```python
from build123d import *

# Parameters (mm, degrees)
SKETCH1_W           = 20
SKETCH1_H           = 3
BOSS_EXTRUDE1_DEPTH = 3


with BuildPart() as part:
    # Sketch1 → Boss-Extrude1 (new body)
    # profile 1 of 3: a face of its own
    with BuildSketch(Plane.XY):
        Polygon((35, 40), (-35, 25), (-38, 25), (-38, 12.5), (-35, 12.5), (-35, -2.5), (-38, -2.5), (-38, -17.5), (-35, -17.5), (-35, -32.5), (-38, -32.5), (-38, -40), (-27.5, -40), (-7.5, -40), (7.5, -40), (27.5, -40), (38, -40), (38, -37.5), (35, -37.5), (35, -22.5), (38, -22.5), (38, -7.5), (35, -7.5), (35, 7.5), (38, 7.5), (38, 22.5), (35, 22.5), (35, 37.5), (38, 37.5), (38, 40), align=None)
        with BuildLine():
            ThreePointArc((-12.5, -28), (-17.5, -33), (-22.5, -28))
            Line((-22.5, -28), (-22.5, 12))
            ThreePointArc((-22.5, 12), (-17.5, 17), (-12.5, 12))
            Line((-12.5, 12), (-12.5, -28))
        make_face(mode=Mode.SUBTRACT)
        with BuildLine():
            ThreePointArc((-5, 17), (0, 22), (5, 17))
            Line((5, 17), (5, -28))
            ThreePointArc((5, -28), (0, -33), (-5, -28))
            Line((-5, -28), (-5, 17))
        make_face(mode=Mode.SUBTRACT)
        with BuildLine():
            ThreePointArc((22.5, -28), (17.5, -33), (12.5, -28))
            Line((12.5, -28), (12.5, 22))
            ThreePointArc((12.5, 22), (17.5, 27), (22.5, 22))
            Line((22.5, 22), (22.5, -28))
        make_face(mode=Mode.SUBTRACT)
    # profile 2 of 3: a face of its own
    with BuildSketch(Plane.XY):
        with Locations((17.5, -41.5)):
            Rectangle(SKETCH1_W, SKETCH1_H)
    # profile 3 of 3: a face of its own
    with BuildSketch(Plane.XY):
        with Locations((-17.5, -41.5)):
            Rectangle(SKETCH1_W, SKETCH1_H)
    extrude(amount=BOSS_EXTRUDE1_DEPTH)


solid = part.part
```
Geometry check sheet. Reference: the model listing, model coordinates, mm. A direction names the side the tool comes from. Give positions to 0.01 mm unless a question says otherwise; leave off trailing zeros. Order: outer loops, then holes, each group sorted by start corner. A loop starts at its lowest first (then second) coordinate and runs counter-clockwise, first axis right, second up.
1. Gauge pin test, flat ends, axial feed: pin 1 Ø1.5 at (y, z) = (5, 2) entering from +X; pin 2 Ø1.5 at (y, z) = (-24, 2) entering from -X; pin 3 Ø0.9 at (x, z) = (34, 1.5) entering from -Y. Record the tip position at first contact, or that the pin passes through.
2. Thickness scan on L1, parallel to X at y = -1, z = 1.45; L2, parallel to X at y = -21, z = 1.05; L3, parallel to X at y = 19.5, z = 1.2. Record the ranges inside material, lowest first.
3. Release check for a two-part mould opening along X. For faces 1 (the face through (-17.6, 17, 1.5)), 2 (the face through (36, -22.5, 1)), 3 (the face through (38, 39, 1)) record: pulls with the +X half, pulls with the -X half, needs draft (parallel to the pull), parting line crosses it, or undercut.
4. Access from +Z, -Z, +X, -X, +Y, -Y to the whole of each face (thin tool, end or side, straight path). Record for faces 4 (the face through (37, 22.5, 1)), 5 (the face through (33, -40, 1)), 6 (the face through (-22.5, -8, 1)).
5. Section check D-D, the plane x = 0. Enter the section's corners in (y, z).
6. Section check C-C, the plane z = 0.7. Give the number of separate pieces and of enclosed holes in the cut face, and give its area (3 significant figures).
7. Section check B-B, the plane x = 17.5. Enter the section's corners in (y, z), and give its area (4 significant figures).
8. Section check A-A, the plane y = -1.5. Enter the section's corners in (x, z).
Values follow:
1. pin 1: stops at x = 35
1. pin 2: stops at x = -35
1. pin 3: stops at y = -40
2. L1: x = -35 to -22.5, -12.5 to -5, 5 to 12.5, 22.5 to 35
2. L2: x = -35 to -22.5, -12.5 to -5, 5 to 12.5, 22.5 to 38
2. L3: x = -38 to -4.33, 4.33 to 12.5, 22.5 to 38
3. face 1: undercut
3. face 2: needs draft
3. face 3: pulls with the +X half
4. face 4: +Z, -Z, +X
4. face 5: +Z, -Z, +X, -Y
4. face 6: +Z, -Z
5. outline: (-40, 0) - (-33, 0) - (-33, 3) - (-40, 3) - close; (22, 0) - (32.5, 0) - (32.5, 3) - (22, 3) - close
6. separate pieces: 1
6. enclosed holes: 3
6. area: 3,820 mm2
7. outline: (-43, 0) - (-33, 0) - (-33, 3) - (-43, 3) - close; (27, 0) - (36.25, 0) - (36.25, 3) - (27, 3) - close
7. area: 57.75 mm2
8. outline: (-35, 0) - (-22.5, 0) - (-22.5, 3) - (-35, 3) - close; (-12.5, 0) - (-5, 0) - (-5, 3) - (-12.5, 3) - close; (5, 0) - (12.5, 0) - (12.5, 3) - (5, 3) - close; (22.5, 0) - (35, 0) - (35, 3) - (22.5, 3) - close
